```python
from build123d import *

# Parameters (mm, degrees)
F3_R     = 26.8
F3_R_2   = 6.7
F4_DEPTH = 2.5
F5_R     = 10.3
F5_R_2   = 9
F6_DEPTH = 1
F7_R     = 0.5
F9_DEPTH = 2


with BuildPart() as f4:
    # F3 (on Top) → F4 (new body)
    with BuildSketch(Plane.XY):
        Circle(F3_R)
        with BuildLine():
            Line((-4.1619996915, -13.4381969615), (-4.1619996915, -17.9131179147))
            Line((-4.1619996915, -17.9131179147), (-4.657580782, -17.9131179147))
            Line((-4.657580782, -17.9131179147), (-4.657580782, -14.7241613326))
            add(Edge.make_bspline(
                [(-4.657580782, -14.7241613326), (-4.657580782, -14.3255417599), (-4.6330955502, -13.9709956042)],
                knots=[0, 0, 0, 1, 1, 1], degree=2))
            add(Edge.make_bspline(
                [(-4.6330955502, -13.9709956042), (-4.6967571528, -14.035636616), (-4.7765790083, -14.1056643788)],
                knots=[0, 0, 0, 1, 1, 1], degree=2))
            add(Edge.make_bspline(
                [(-4.7765790083, -14.1056643788), (-4.8564008637, -14.1756921416), (-5.5047698003, -14.7026143287)],
                knots=[0, 0, 0, 1, 1, 1], degree=2))
            Line((-5.5047698003, -14.7026143287), (-5.7741073494, -14.3539446287))
            Line((-5.7741073494, -14.3539446287), (-4.5900015424, -13.4381969615))
            Line((-4.5900015424, -13.4381969615), (-4.1619996915, -13.4381969615))
        make_face(mode=Mode.SUBTRACT)
        with BuildLine():
            add(Edge.make_bspline(
                [(-0.0484807588, -13.6727654816), (0.3129212617, -13.9709956042), (0.3129212617, -14.4910619264)],
                knots=[0, 0, 0, 1, 1, 1], degree=2))
            add(Edge.make_bspline(
                [(0.3129212617, -14.4910619264), (0.3129212617, -14.9200431866), (0.072476286, -15.1923189635)],
                knots=[0, 0, 0, 1, 1, 1], degree=2))
            add(Edge.make_bspline(
                [(0.072476286, -15.1923189635), (-0.1679686898, -15.4645947405), (-0.6087028611, -15.5566592118)],
                knots=[0, 0, 0, 1, 1, 1], degree=2))
            Line((-0.6087028611, -15.5566592118), (-0.6087028611, -15.5811444436))
            add(Edge.make_bspline(
                [(-0.6087028611, -15.5811444436), (-0.0700277628, -15.6477442739), (0.1900053983, -15.9234479833)],
                knots=[0, 0, 0, 1, 1, 1], degree=2))
            add(Edge.make_bspline(
                [(0.1900053983, -15.9234479833), (0.4500385594, -16.1991516928), (0.4500385594, -16.6457623197)],
                knots=[0, 0, 0, 1, 1, 1], degree=2))
            add(Edge.make_bspline(
                [(0.4500385594, -16.6457623197), (0.4500385594, -17.2853165728), (0.0063661603, -17.6300686358)],
                knots=[0, 0, 0, 1, 1, 1], degree=2))
            add(Edge.make_bspline(
                [(0.0063661603, -17.6300686358), (-0.4373062389, -17.9748206987), (-1.2541335698, -17.9748206987)],
                knots=[0, 0, 0, 1, 1, 1], degree=2))
            add(Edge.make_bspline(
                [(-1.2541335698, -17.9748206987), (-1.6096591347, -17.9748206987), (-1.9049510295, -17.9209531889)],
                knots=[0, 0, 0, 1, 1, 1], degree=2))
            add(Edge.make_bspline(
                [(-1.9049510295, -17.9209531889), (-2.2002429243, -17.867085679), (-2.4783951569, -17.7329066091)],
                knots=[0, 0, 0, 1, 1, 1], degree=2))
            Line((-2.4783951569, -17.7329066091), (-2.4783951569, -17.2490784299))
            add(Edge.make_bspline(
                [(-2.4783951569, -17.2490784299), (-2.1875106038, -17.3930515925), (-1.8584290892, -17.4679764016)],
                knots=[0, 0, 0, 1, 1, 1], degree=2))
            add(Edge.make_bspline(
                [(-1.8584290892, -17.4679764016), (-1.5293475746, -17.5429012108), (-1.2355247937, -17.5429012108)],
                knots=[0, 0, 0, 1, 1, 1], degree=2))
            add(Edge.make_bspline(
                [(-1.2355247937, -17.5429012108), (-0.0759042184, -17.5429012108), (-0.0759042184, -16.6340094085)],
                knots=[0, 0, 0, 1, 1, 1], degree=2))
            add(Edge.make_bspline(
                [(-0.0759042184, -16.6340094085), (-0.0759042184, -15.8191408961), (-1.3550127246, -15.8191408961)],
                knots=[0, 0, 0, 1, 1, 1], degree=2))
            Line((-1.3550127246, -15.8191408961), (-1.795746896, -15.8191408961))
            Line((-1.795746896, -15.8191408961), (-1.795746896, -15.3823243618))
            Line((-1.795746896, -15.3823243618), (-1.349136269, -15.3823243618))
            add(Edge.make_bspline(
                [(-1.349136269, -15.3823243618), (-0.826131719, -15.3823243618), (-0.5200663222, -15.1511837742)],
                knots=[0, 0, 0, 1, 1, 1], degree=2))
            add(Edge.make_bspline(
                [(-0.5200663222, -15.1511837742), (-0.2140009254, -14.9200431866), (-0.2140009254, -14.5096707026)],
                knots=[0, 0, 0, 1, 1, 1], degree=2))
            add(Edge.make_bspline(
                [(-0.2140009254, -14.5096707026), (-0.2140009254, -14.1825480065), (-0.4387753528, -13.995480836)],
                knots=[0, 0, 0, 1, 1, 1], degree=2))
            add(Edge.make_bspline(
                [(-0.4387753528, -13.995480836), (-0.6635497802, -13.8084136655), (-1.0494370325, -13.8084136655)],
                knots=[0, 0, 0, 1, 1, 1], degree=2))
            add(Edge.make_bspline(
                [(-1.0494370325, -13.8084136655), (-1.3432598134, -13.8084136655), (-1.6032929745, -13.8882355209)],
                knots=[0, 0, 0, 1, 1, 1], degree=2))
            add(Edge.make_bspline(
                [(-1.6032929745, -13.8882355209), (-1.8633261356, -13.9680573764), (-2.1973046965, -14.1825480065)],
                knots=[0, 0, 0, 1, 1, 1], degree=2))
            Line((-2.1973046965, -14.1825480065), (-2.4539099252, -13.8397547621))
            add(Edge.make_bspline(
                [(-2.4539099252, -13.8397547621), (-2.1786959204, -13.6223259042), (-1.8192527184, -13.4984306316)],
                knots=[0, 0, 0, 1, 1, 1], degree=2))
            add(Edge.make_bspline(
                [(-1.8192527184, -13.4984306316), (-1.4598095165, -13.374535359), (-1.0611899437, -13.374535359)],
                knots=[0, 0, 0, 1, 1, 1], degree=2))
            add(Edge.make_bspline(
                [(-1.0611899437, -13.374535359), (-0.4098827794, -13.374535359), (-0.0484807588, -13.6727654816)],
                knots=[0, 0, 0, 1, 1, 1], degree=2))
        make_face(mode=Mode.SUBTRACT)
        Circle(F3_R_2, mode=Mode.SUBTRACT)
        with BuildLine():
            add(Edge.make_bspline(
                [(1.3848847073, -17.9057723452), (1.2825364387, -17.8093005321), (1.2825364387, -17.5889334464)],
                knots=[0, 0, 0, 1, 1, 1], degree=2))
            add(Edge.make_bspline(
                [(1.2825364387, -17.5889334464), (1.2825364387, -17.3832574998), (1.3760700239, -17.2779710033)],
                knots=[0, 0, 0, 1, 1, 1], degree=2))
            add(Edge.make_bspline(
                [(1.3760700239, -17.2779710033), (1.4696036092, -17.1726845068), (1.6439384592, -17.1726845068)],
                knots=[0, 0, 0, 1, 1, 1], degree=2))
            add(Edge.make_bspline(
                [(1.6439384592, -17.1726845068), (1.821211537, -17.1726845068), (1.9206215779, -17.2779710033)],
                knots=[0, 0, 0, 1, 1, 1], degree=2))
            add(Edge.make_bspline(
                [(1.9206215779, -17.2779710033), (2.0200316187, -17.3832574998), (2.0200316187, -17.5889334464)],
                knots=[0, 0, 0, 1, 1, 1], degree=2))
            add(Edge.make_bspline(
                [(2.0200316187, -17.5889334464), (2.0200316187, -17.7877535282), (1.9191524639, -17.8949988432)],
                knots=[0, 0, 0, 1, 1, 1], degree=2))
            add(Edge.make_bspline(
                [(1.9191524639, -17.8949988432), (1.8182733092, -18.0022441582), (1.6439384592, -18.0022441582)],
                knots=[0, 0, 0, 1, 1, 1], degree=2))
            add(Edge.make_bspline(
                [(1.6439384592, -18.0022441582), (1.487232976, -18.0022441582), (1.3848847073, -17.9057723452)],
                knots=[0, 0, 0, 1, 1, 1], degree=2))
        make_face(mode=Mode.SUBTRACT)
        Polygon((5.9435451531, -16.4224570062), (5.9435451531, -16.8847381815), (5.2795056682, -16.8847381815), (5.2795056682, -17.9131179147), (4.7927392612, -17.9131179147), (4.7927392612, -16.8847381815), (2.616491864, -16.8847381815), (2.616491864, -16.4410657824), (4.7408305699, -13.4137117298), (5.2795056682, -13.4137117298), (5.2795056682, -16.4224570062), align=None, mode=Mode.SUBTRACT)
    extrude(amount=F4_DEPTH)

    # F5 (on face) → F6 (join)
    with BuildSketch(Plane.XY.offset(2.5)):
        Circle(F5_R)
        Circle(F5_R_2, mode=Mode.SUBTRACT)
    extrude(amount=F6_DEPTH)

    # F7
    f7_edges = [f4.edges().sort_by_distance(p)[0] for p in [
        (-10.3, 0, 3.5),
    ]]
    fillet(f7_edges, radius=F7_R)

    # F8 (on face) → F9 (join)
    with BuildSketch(Plane(origin=(0, 0, 0), x_dir=(1, 0, 0), z_dir=(0, 0, -1))):
        with BuildLine():
            Line((-5.2854986866, 10.6844577384), (-8.5731837258, 4.7476858367))
            ThreePointArc((-8.5731837258, 4.7476858367), (0, -9.8), (8.5731837258, 4.7476858367))
            Line((8.5731837258, 4.7476858367), (5.2854986866, 10.6844577384))
            ThreePointArc((5.2854986866, 10.6844577384), (4.9183956817, 11.0615270566), (4.4106840207, 11.2))
            Line((4.4106840207, 11.2), (-4.4106840207, 11.2))
            ThreePointArc((-4.4106840207, 11.2), (-4.9183956817, 11.0615270566), (-5.2854986866, 10.6844577384))
        make_face()
        with BuildLine():
            ThreePointArc((7.4359246601, 4.1178907767), (0, -8.5), (-7.4359246601, 4.1178907767))
            Line((-7.4359246601, 4.1178907767), (-4.3766385702, 9.6422288692))
            ThreePointArc((-4.3766385702, 9.6422288692), (-4.1930870677, 9.8307635283), (-3.9392312372, 9.9))
            Line((-3.9392312372, 9.9), (3.9392312372, 9.9))
            ThreePointArc((3.9392312372, 9.9), (4.1930870677, 9.8307635283), (4.3766385702, 9.6422288692))
            Line((4.3766385702, 9.6422288692), (7.4359246601, 4.1178907767))
        make_face(mode=Mode.SUBTRACT)
    extrude(amount=F9_DEPTH)


solid = f4.part
```
Here's how the part is built. I have some questions about the finished solid (model axes, mm). A direction names the side the tool comes from. Round coordinates to 2 decimals unless told otherwise and drop trailing zeros. Write each loop counter-clockwise with the first axis right and the second up, starting at its lowest first coordinate (ties: lowest second). Pieces come first, ordered by that corner, then holes. Notation, with made-up numbers: M 60,-12 L 115,-12 A6 ccw 115,-2 Z; hole C 21,44.5 d9. An arc over 180 degrees is marked long. Answer as CSV lines item,"result". Start each with the question number.
1. Suppose I cut it at B-B on y = 17.5. Write out the boundary of the cut face in (x, z).
2. Thinking about a two-plate mould opening in X: for faces 1 (the flat face through (-6.906, -7.758, -0.986)), 2 (the flat face through (0, -11.2, -1)), 3 (the cylindrical face through (9.824, 3.094, 2.746)), 4 (the flat face through (0, 7, 2.5)), which applies, released by +X, released by -X, zero draft, split by the parting line, or undercut?
3. I'm going to push flat-ended pins straight in: pin 1 Ø4 at (x, y) = (19, -13) entering from +Z; pin 2 Ø1.1 at (y, z) = (-17.5, 1) entering from -X; pin 3 Ø2 at (y, z) = (-1, -0.5) entering from -X. Where does each tip first touch, or does it pass through?
4. On a 3-axis mill with a long thin cutter (end or side, diameter ignored), from which of +Z, -Z, +X, -X, +Y, -Y can I reach the whole of each face in a straight line? I mean faces 5 (the flat face through (4, -16.885, 1)), 6 (the flat face through (0, -7, 0)), 7 (the flat face through (6.952, -7.675, -0.986)). Say none if no direction works.
5. I need wall thicknesses on probe 1 along Y at (x, z) = (0, -0.65); probe 2 along Y at (x, z) = (0, 3.1); probe 3 along X at (y, z) = (0, -0.5). Which ranges of each line are inside material? Lowest first, please.
6. Suppose I cut it at A-A on y = 0. Write out the boundary of the cut face in (x, z).
Check result:
1,outline,"M -20.3,0 L 20.3,0 L 20.3,2.5 L -20.3,2.5 Z"
2,face 1,"released by -X"
2,face 2,"zero draft"
2,face 3,"split by the parting line"
2,face 4,"undercut"
3,pin 1,"stops at z = 2.5"
3,pin 2,"stops at x = -20.76"
3,pin 3,"stops at x = -26.8"
4,face 5,"+Z, -Z"
4,face 6,"-Z"
4,face 7,"-Z, +X, -Y"
5,probe 1,"y = -11.2 to -9.9, 8.5 to 9.8"
5,probe 2,"y = -10.29 to -9, 9 to 10.29"
5,probe 3,"x = -9.8 to -8.5, 8.5 to 9.8"
6,outline,"M -26.8,0 L -9.8,0 L -9.8,-2 L -8.5,-2 L -8.5,0 L -6.7,0 L -6.7,2.5 L -9,2.5 L -9,3.5 L -9.8,3.5 A0.5 ccw -10.3,3 L -10.3,2.5 L -26.8,2.5 Z; M 6.7,0 L 8.5,0 L 8.5,-2 L 9.8,-2 L 9.8,0 L 26.8,0 L 26.8,2.5 L 10.3,2.5 L 10.3,3 A0.5 ccw 9.8,3.5 L 9,3.5 L 9,2.5 L 6.7,2.5 Z"
